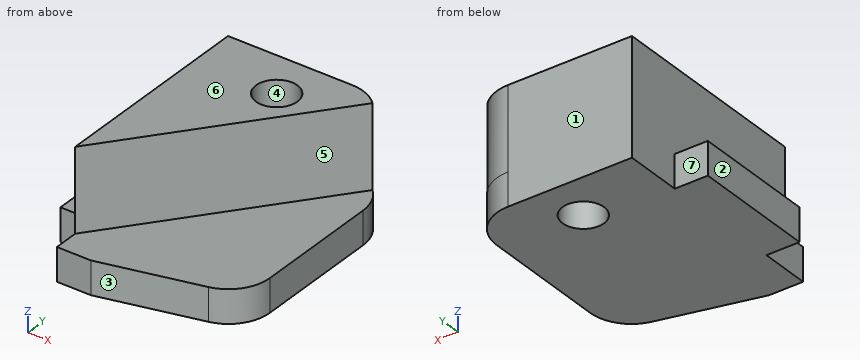
```python
from build123d import *

# Parameters (mm, degrees)
SKETCH_1_R      = 2.5
EXTRUDE_1_DEPTH = 4
FILLET_1_R      = 5
SKETCH_2_R      = 2.5
EXTRUDE_2_DEPTH = 10


with BuildPart() as part:
    # ｽｹｯﾁ1 → ﾎﾞｽ - 押し出し1 (new body)
    with BuildSketch(Plane.XY):
        Polygon((0, 15), (0, 0), (4, 0), (4, -6), (8.110763801, -6), (24, -2.18322685), (24, 22), (4, 22), (4, 15), align=None)
        with Locations((14, 16.41)):
            Circle(SKETCH_1_R, mode=Mode.SUBTRACT)
    extrude(amount=EXTRUDE_1_DEPTH)

    # ﾌｨﾚｯﾄ1
    fillet_1_edges = [part.edges().sort_by_distance(p)[0] for p in [
        (24, 22, 2),
        (24, -2.18322685, 2),
    ]]
    fillet(fillet_1_edges, radius=FILLET_1_R)

    # ｽｹｯﾁ2 → ﾎﾞｽ - 押し出し2 (add)
    with BuildSketch(Plane.XY.offset(4)):
        with BuildLine():
            Line((4, 0), (4, -3))
            Line((4, -3), (22.535533906, 20.535533906))
            ThreePointArc((22.535533906, 20.535533906), (20.913417162, 21.619397663), (19, 22))
            Line((19, 22), (4, 22))
            Line((4, 22), (4, 15))
            Line((4, 15), (4, 0))
        make_face()
        with Locations((14, 16.41)):
            Circle(SKETCH_2_R, mode=Mode.SUBTRACT)
    extrude(amount=EXTRUDE_2_DEPTH)


solid = part.part
```
Here's how the part is built. I have some questions about the finished solid (model axes, mm). Face numbers are marked on the shaded views. A direction names the side the tool comes from. Round coordinates to 2 decimals unless told otherwise and drop trailing zeros. Write each loop counter-clockwise with the first axis right and the second up, starting at its lowest first coordinate (ties: lowest second). Pieces come first, ordered by that corner, then holes.
Q1. If we section it at A-A on y = 16.41: Write out the boundary of the cut face in (x, z), plus the area to 3 significant figures.
Q2. Will these pins go through, and if not, where does the flat tip stop? P1, Ø1, axis at x = 20.5, y = -2.5, coming from the +Z side; P2, Ø1.2, axis at x = 2, z = 2.5, coming from the -Y side; P3, Ø3, axis at x = 10, z = 2, coming from the -Y side.
Q3. If we section it at B-B on z = 11.25: Write out the boundary of the cut face in (x, y).
Q4. If we section it at C-C on x = 14: Write out the boundary of the cut face in (y, z).
Q5. Please list where these lines run through material, in increasing order: probe 1 along Y at (x, z) = (7.75, 13); probe 2 along Z at (x, y) = (19.75, 3.25); probe 3 along X at (y, z) = (14.25, 10).
Q6. Which directions (+Z, -Z, +X, -X, +Y, -Y) give clear straight access to the entire face, cutting with the end or side of a thin tool? Please do the marked faces 5, 6 and 7.
Q7. If we mould it in two halves opening along X, with no side actions, what happens to the marked faces 1, 2, 3 and 4? For each: +X half, -X half, draft (parallel to the pull), parting line (faces both ways), or undercut.
Q8. If we section it at D-D on y = 2.5: Write out the boundary of the cut face in (x, z), plus the area to 3 significant figures.
Answer below:
1. outline: (4, 0) - (11.5, 0) - (11.5, 14) - (4, 14) - close; (16.5, 0) - (24, 0) - (24, 4) - (19.29, 4) - (19.29, 14) - (16.5, 14) - close
1. area: 163 mm2
2. P1: stops at z = 4
2. P2: stops at y = 0
2. P3: stops at y = -5.91
3. outline: (4, -3) - (22.54, 20.54) arc R5 ccw to (19, 22) - (4, 22) - close; hole circle Ø5 at (14, 16.41)
4. outline: (-4.59, 0) - (13.91, 0) - (13.91, 14) - (9.7, 14) - (9.7, 4) - (-4.59, 4) - close; (18.91, 0) - (22, 0) - (22, 14) - (18.91, 14) - close
5. probe 1: y = 1.76 to 22
5. probe 2: z = 0 to 4
5. probe 3: x = 4 to 12.74, 15.26 to 17.59
6. face 5: +Z, +X, -Y
6. face 6: +Z, +X, -X, +Y, -Y
6. face 7: +Z, -Z, -X, +Y
7. face 1: draft
7. face 2: -X half
7. face 3: +X half
7. face 4: undercut
8. outline: (0, 0) - (24, 0) - (24, 4) - (8.33, 4) - (8.33, 14) - (4, 14) - (4, 4) - (0, 4) - close
8. area: 139 mm2
